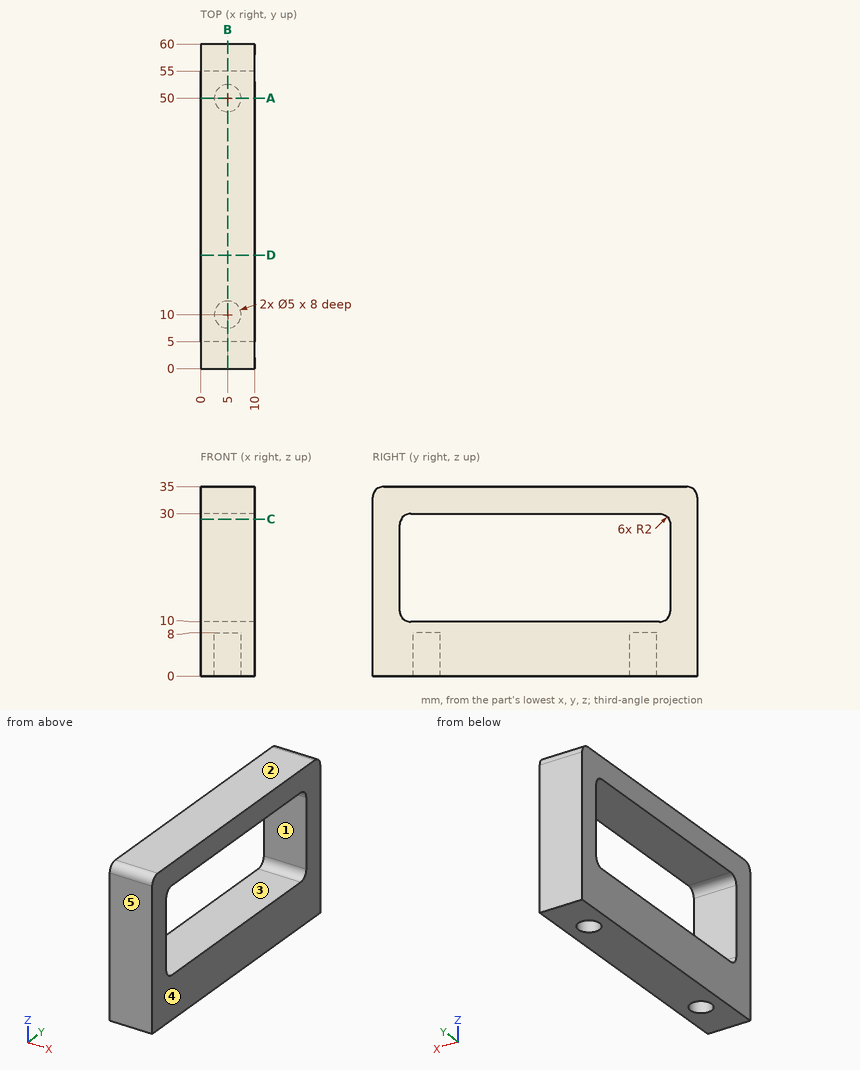
The figure shows three views and two pictorial views of one solid part (mm, origin at its lowest corner). Answer the questions. A direction names the side the tool comes from. Give positions to 0.01 mm unless a question says otherwise; leave off trailing zeros. Order: outer loops, then holes, each group sorted by start corner. A loop starts at its lowest first (then second) coordinate and runs counter-clockwise, first axis right, second up. Notation, with made-up numbers: (86, 86) - (111, 86) arc R25 ccw to (111, 116) - close; hole circle Ø9 at (-6.5, 36). An arc over 180 degrees is marked (long way). Answer as CSV lines item,"result".
Q1. A cutting plane is placed at A-A, the plane y = 50. Determine the outline of the cut face in (x, z).
Answer key:
outline,"(0, 0) - (2.5, 0) - (2.5, 8) - (7.5, 8) - (7.5, 0) - (10, 0) - (10, 10) - (0, 10) - close; (0, 30) - (10, 30) - (10, 35) - (0, 35) - close"
Q2. A cutting plane is placed at B-B, the plane x = 5. Determine the outline of the cut face in (y, z), and give its area (3 significant figures).
Answer key:
outline,"(0, 0) - (7.5, 0) - (7.5, 8) - (12.5, 8) - (12.5, 0) - (47.5, 0) - (47.5, 8) - (52.5, 8) - (52.5, 0) - (60, 0) - (60, 33) arc R2 ccw to (58, 35) - (2, 35) arc R2 ccw to (0, 33) - close; hole (5, 12) arc R2 ccw to (7, 10) - (53, 10) arc R2 ccw to (55, 12) - (55, 28) arc R2 ccw to (53, 30) - (7, 30) arc R2 ccw to (5, 28) - close"
area,"1,020 mm^2"
Q3. Determine the mould class of the marked faces 3, 4 and 5 for opening direction Y: pulls with the +Y half, pulls with the -Y half, needs draft (parallel to the pull), parting line crosses it, or undercut.
Answer key:
face 3,"undercut"
face 4,"needs draft"
face 5,"pulls with the -Y half"
Q4. Straight lines are drawn through the part: L1, parallel to Y at x = 5, z = 6; L2, parallel to X at y = 50, z = 4.5; L3, parallel to Y at x = 8.25, z = 24.5. For each, find the intervals that lie inside material, in ascending order.
Answer key:
L1,"y = 0 to 7.5, 12.5 to 47.5, 52.5 to 60"
L2,"x = 0 to 2.5, 7.5 to 10"
L3,"y = 0 to 5, 55 to 60"
Q5. A cutting plane is placed at D-D, the plane y = 21. Determine the outline of the cut face in (x, z).
Answer key:
outline,"(0, 0) - (10, 0) - (10, 10) - (0, 10) - close; (0, 30) - (10, 30) - (10, 35) - (0, 35) - close"
Q6. Which of the six approach directions +Z, -Z, +X, -X, +Y, -Y give full straight-line access (tool end or side, diameter ignored) to the marked faces 1 and 2?
Answer key:
face 1,"+X, -X"
face 2,"+Z, +X, -X, +Y, -Y"
Q7. A cutting plane is placed at C-C, the plane z = 29. Determine the outline of the cut face in (x, y).
Answer key:
outline,"(0, 0) - (10, 0) - (10, 5.27) - (0, 5.27) - close; (0, 54.73) - (10, 54.73) - (10, 60) - (0, 60) - close"
Q8. Each of these flat-tipped pins is pushed along its axis until it touches: pin 1 Ø5 at (y, z) = (18, 26) entering from -X; pin 2 Ø3 at (x, y) = (5, 10) entering from -Z. Where does it stop, or does it pass through?
Answer key:
pin 1,"passes through"
pin 2,"stops at z = 8"
